Autodesk Inventor part; units mm, degrees
ref_plane "YZ Plane" through (0, 0, 0) normal (1, 0, 0) x (0, 1, 0)
ref_plane "XZ Plane" through (0, 0, 0) normal (0, 1, 0) x (-1, 0, 0)
ref_plane "XY Plane" through (0, 0, 0) normal (0, 0, 1) x (1, 0, 0)
sketch "Sketch1" plane through (0, 0, 0) normal (0, 0, 1) x (1, 0, 0)
  line L0 (-73.2051, 41.2219) -> (-136.7051, 41.2219)
  line L1 (-143.0551, 47.5719) -> (-143.0551, 98.3719)
  line L2 (-143.0551, 98.3719) -> (-66.8551, 98.3719)
  line L3 (-66.8551, 98.3719) -> (-66.8551, 47.5719)
  line L4 (-143.0551, 47.5719) -> (-136.7051, 41.2219)
  line L5 (-73.2051, 41.2219) -> (-66.8551, 47.5719)
  point P0 (0, 0)
  point P1 (-66.8551, 41.2219)
  point P2 (-143.0551, 41.2219)
  point P3 (-117.6551, 41.2219)
  point P4 (-143.0551, 66.6219)
  point P5 (-66.8551, 72.9719)
  point P6 (-92.2551, 41.2219)
  point P7 (-143.0551, 41.2219)
  point P8 (-66.8551, 41.2219)
  dimension "d0" = 76.2
  dimension "d1" = 57.15
  dimension "d10" = 6.35
  dimension "d11" = 6.35
  dimension "d12" = 6.35
extrude "Extrusion1" add sketch "Sketch1" along normal blind 6.35
sketch "Sketch2" plane through (0, 0, 6.35) normal (0, 0, 1) x (1, 0, 0)
  line L0 (-130.3551, 77.0986) -> (-130.3551, 56.1453)
  line L1 (-130.3551, 66.6219) -> (-98.3601, 66.6219) construction
  arc A0 (-120.0565, 65.1716) -> (-124.5928, 66.6219) centre (-122.0928, 66.6219) ccw
  line L2 (-124.5928, 66.6219) -> (-120.0565, 65.1716)
  point P0 (0, 0)
  dimension "d4" = 5
extrude "Extrusion2" [suppressed]
sketch "Sketch3" plane through (0, 0, 0) normal (0, 0, -1) x (-1, 0, 0)
  arc A0 (124.5928, 66.6219) -> (120.0565, 65.1716) centre (122.0928, 66.6219) ccw
  line L0 (124.5928, 66.6219) -> (120.0565, 65.1716)
  circle A1 centre (122.0928, 66.6219) radius 11
  point P0 (0, 0)
extrude "Extrusion3" [suppressed]
sketch "Sketch4" plane through (0, 0, 0) normal (0, 0, -1) x (-1, 0, 0)
  line L0 (143.0551, 92.0219) -> (133.3409, 92.0219) construction
  line L1 (143.0551, 85.6719) -> (133.3409, 85.6719) construction
  line L2 (143.0551, 85.6719) -> (143.0551, 98.3719) construction
  line L3 (35.1051, 88.8469) -> (143.0551, 88.8469) construction
  circle A0 centre (77.2251, 88.8469) radius 1.8542
  circle A1 centre (131.4867, 88.8469) radius 1.8542
  line L4 (133.3409, 92.0219) -> (133.3409, 85.6719)
  point P0 (0, 0)
  dimension "d15" = 3.7084
  dimension "d16" = 3.7084
extrude "Extrusion4" cut sketch "Sketch4" against normal through all
sketch "Sketch5" plane through (0, 0, 0) normal (0, 0, -1) x (-1, 0, 0)
  circle A0 centre (122.6066, 75.5662) radius 1.5875
  circle A1 centre (131.037, 66.1081) radius 1.5875
  circle A2 centre (121.5789, 57.6777) radius 1.5875
  circle A3 centre (113.1485, 67.1358) radius 1.5875
  point P0 (0, 0)
extrude "Extrusion5" [suppressed]
sketch "Sketch6" plane through (0, 0, 0) normal (0, 0, -1) x (-1, 0, 0)
  circle A0 centre (119.3278, 71.4063) radius 11
  point P0 (0, 0)
extrude "Extrusion6" cut sketch "Sketch6" against normal through all
sketch "Sketch7" plane through (0, 0, 6.35) normal (0, 0, 1) x (1, 0, 0)
  line L0 (-91.6559, 92.0219) -> (-117.0559, 92.0219)
  line L1 (-117.0559, 85.6719) -> (-91.6559, 85.6719)
  line L2 (-91.6559, 85.6719) -> (-91.6559, 92.0219)
  line L3 (-117.0559, 92.0219) -> (-117.0559, 85.6719)
  point P0 (0, 0)
extrude "Extrusion7" cut sketch "Sketch7" against normal through all
properties part number "projectorMountOppositeSide_RB01" material "Wood (Oak)"
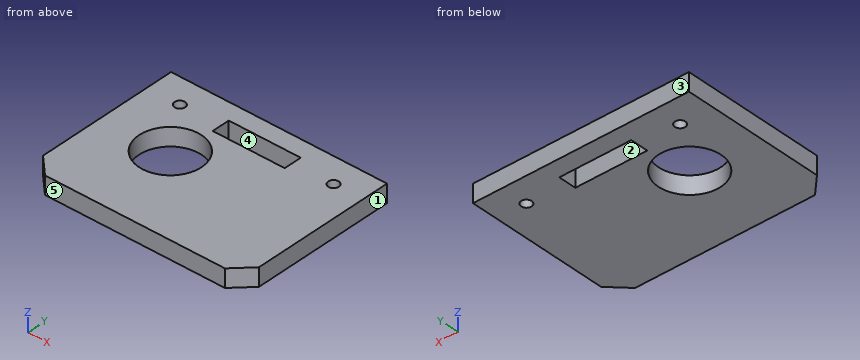
Here's how the part is built. I have some questions about the finished solid (model axes, mm). Face numbers are marked on the shaded views. A direction names the side the tool comes from. Give positions to 0.01 mm unless a question says otherwise; leave off trailing zeros. Loops run counter-clockwise (first coordinate to the right, second up) from the corner with the lowest first, then second, coordinate; pieces in that order, holes last. Notation, with made-up numbers: M -5.5,57 L 50.5,57 A19 cw 50.5,65 Z; hole C 50.5,89 d9. An arc over 180 degrees is marked long. Use one line per item in the form item = value. Start each with the question number.
Q1. I need wall thicknesses on line 1 along X through (y, z) = (89, 5); line 2 along Y through (x, z) = (-119.5, 4.5); line 3 along Y through (x, z) = (-99.5, 2). Which ranges of each line are inside material? Lowest first, please.
Q2. If we section it at A-A (x = -104): Write out the boundary of the cut face in (y, z), then the cut area to 3 significant figures.
Q3. Thinking about a two-plate mould opening in Y: for the marked faces 3, 4 and 5, which applies, +Y half, -Y half, draft (parallel to the pull), parting line (faces both ways), or undercut?
Q4. Which directions (+Z, -Z, +X, -X, +Y, -Y) give clear straight access to the entire face, cutting with the end or side of a thin tool? Please do the marked faces 1 and 2.
Q5. If we section it at D-D (x = -116): Write out the boundary of the cut face in (y, z).
Q6. If we section it at B-B (y = 68.5): Write out the boundary of the cut face in (x, z).
Q7. If we section it at C-C (z = 3): Write out the boundary of the cut face in (x, y).
Taken from the geometry:
q1.line_1 = -143.06 to -133.33, -129.64 to -117.06, -91.66 to -79.07, -75.38 to -66.86
q1.line_2 = 41.22 to 60.41, 82.4 to 98.37
q1.line_3 = 41.22 to 85.67, 92.02 to 98.37
q2.outline = M 41.22,0 L 85.67,0 L 85.67,6.35 L 41.22,6.35 Z; M 92.02,0 L 98.37,0 L 98.37,6.35 L 92.02,6.35 Z
q2.area = 323 mm^2
q3.face_3 = +Y half
q3.face_4 = undercut
q3.face_5 = -Y half
q4.face_1 = +Z, -Z, +X, +Y, -Y
q4.face_2 = +Z, -Z
q5.outline = M 41.22,0 L 60.92,0 L 60.92,6.35 L 41.22,6.35 Z; M 81.89,0 L 85.67,0 L 85.67,6.35 L 81.89,6.35 Z; M 92.02,0 L 98.37,0 L 98.37,6.35 L 92.02,6.35 Z
q6.outline = M -143.06,0 L -129.94,0 L -129.94,6.35 L -143.06,6.35 Z; M -108.72,0 L -66.86,0 L -66.86,6.35 L -108.72,6.35 Z
q7.outline = M -143.06,47.57 L -136.71,41.22 L -73.21,41.22 L -66.86,47.57 L -66.86,98.37 L -143.06,98.37 Z; hole C -131.49,88.85 d3.71; hole C -119.33,71.41 d22; hole M -117.06,85.67 L -91.66,85.67 L -91.66,92.02 L -117.06,92.02 Z; hole C -77.23,88.85 d3.71
